For this review, take the finished solid that the model builds, in its own axes (mm). A direction names the side the tool comes from. Round coordinates to 2 decimals unless told otherwise and drop trailing zeros. Loops run counter-clockwise (first coordinate to the right, second up) from the corner with the lowest first, then second, coordinate; pieces in that order, holes last.
1) Take a section at B-B (y = 11.5). State the section outline as (x, z) points, then the cut area to 3 significant figures.
2) Insertion check: pin 1 (1.5 mm diameter, centred on x = 15.5, z = 12, fed in from -Y); pin 2 (4 mm diameter, centred on x = 34.5, y = 21, fed in from +Z); pin 3 (2 mm diameter, centred on x = 10.5, z = 24, fed in from +Y); pin 4 (7 mm diameter, centred on x = 31.02, z = 4, fed in from +Y). Each pin has a flat end and moves straight along its axis. Give the tip position at first contact, or say it passes through.
3) Take a section at C-C (z = 27). State the section outline as (x, y) points, then the cut area to 3 significant figures.
4) Tool access review of faces 4 (the flat face through (20, 58, 9)), 5 (the flat face through (19, 26, 22)), 6 (the flat face through (6.041, 31, 4)), 7 (the flat face through (9, 31, 24)): name each direction out of +Z, -Z, +X, -X, +Y, -Y from which nothing blocks a thin tool from reaching the whole face with its end or side.
5) Take a section at D-D (x = 34). State the section outline as (y, z) points.
6) Take a section at A-A (y = 26.5). Give the number of separate pieces and of enclosed holes in the cut face, then the cut area to 3 significant figures.
7) Mouldability with a two-part tool opening along X and no side actions: class faces 1 (the flat face through (7, 26, 22)), 2 (the flat face through (11, 27, 22)), 3 (the flat face through (21, 27, 34.408)) as pulls with the +X half, pulls with the -X half, needs draft (parallel to the pull), parting line crosses it, or undercut.
8) Wall thickness on L1, parallel to Z at x = 36, y = 6.5; L2, parallel to X at y = 26.5, z = 17; L3, parallel to Y at x = 1, z = 5: over which ranges is each line inside the solid? List them lowest first.
Autodesk Inventor part; units mm, degrees
ref_plane "YZ Plane" through (0, 0, 0) normal (1, 0, 0) x (0, 1, 0)
ref_plane "XZ Plane" through (0, 0, 0) normal (0, 1, 0) x (-1, 0, 0)
ref_plane "XY Plane" through (0, 0, 0) normal (0, 0, 1) x (1, 0, 0)
sketch "Sketch1" plane through (0, 0, 0) normal (0, 1, 0) x (-1, 0, 0)
  line L0 (-6.023191, 2.500092) -> (-6.023191, 5.500092) construction
  line L1 (-6.023191, 4.000092) -> (-13.023191, 4.000092) construction
  line L2 (-6.041071, 8.03122) -> (-6.041071, 4.000092)
  line L3 (-6.041071, -0.031037) -> (-13.023191, -4.062166)
  line L4 (-13.023191, -4.062166) -> (-20.005311, -0.031037)
  line L5 (-20.005311, -0.031037) -> (-20.005311, 8.03122)
  line L6 (-20.005311, 8.03122) -> (-13.023191, 12.062349)
  line L7 (-13.023191, 12.062349) -> (-6.041071, 8.03122)
  line L8 (-22.03646, 9.203905) -> (-22.03646, -1.203722)
  line L9 (-22.03646, -1.203722) -> (-13.023191, -6.407535)
  line L10 (-13.023191, 14.407718) -> (-22.03646, 9.203905)
  line L11 (-13.023191, 4.000092) -> (-31.023191, 4.000092) construction
  circle A0 centre (-31.023191, 4.000092) radius 7.5
  line L12 (-13.023191, -6.407535) -> (-30.97685, -6.407535)
  line L13 (-30.97685, -6.407535) -> (-30.97685, -3.499765)
  line L14 (-30.97685, 11.499948) -> (-30.97685, 14.407718)
  line L15 (-30.97685, 14.407718) -> (-13.023191, 14.407718)
  circle A1 centre (-13.023191, 4.000092) radius 4.5
  line L16 (-30.97685, 11.499988) -> (-30.97685, 14.407718)
  line L17 (-30.97685, -3.500012) -> (-30.97685, -6.407535)
  line L18 (-13.023191, -4.062166) -> (-13.023191, -6.407535)
  line L19 (-13.023191, 12.062349) -> (-13.023191, 14.407718)
  line L20 (-6.041071, 4.000092) -> (-6.041071, -0.031037)
  line L21 (-13.023191, 14.407718) -> (0, 14.407718)
  line L22 (0, 39) -> (0, 0)
  line L23 (0, 14.407718) -> (0, 8.03122)
  line L24 (0, 8.03122) -> (-6.041071, 8.03122)
  line L25 (0, 0) -> (-6, 0)
  line L26 (-13.023191, -6.407535) -> (-2, 0)
  line L27 (-2, 0) -> (-2, 8.03122)
  line L28 (-2, 0) -> (0, 0)
  line L29 (0, 8.03122) -> (0, 0)
  circle A2 centre (-31.023191, 4.000092) radius 4
  line L30 (-30.97685, -3.500012) -> (-38.523191, -3.500012)
  line L31 (-38.523191, -3.500012) -> (-38.523191, -6.407535)
  line L32 (-38.523191, -6.407535) -> (-30.97685, -6.407535)
  line L33 (-30.97685, -6.407535) -> (-30.97685, -3.500012)
  line L34 (-30.97685, 14.407718) -> (-38.523191, 14.407718)
  line L35 (-38.523191, 14.407718) -> (-38.523191, 11.499988)
  line L36 (-38.523191, 11.499988) -> (-30.97685, 11.499988)
  line L37 (-30.97685, 11.499988) -> (-30.97685, 14.407718)
  line L38 (0, 26) -> (-15, 26) construction
  point P0 (0, 31)
  dimension "d0" = 7
  dimension "d1" = 18
  dimension "d2" = 15
  dimension "d3" = 9
  dimension "d4" = 8
  dimension "d6" = 15
extrude "Extrusion1" add sketch "Sketch1" along normal blind 58 contours L24 L27 L26 L18 L3 L20 L2 | L7 L19 L21 L22 L24 | L6 L5 L4 L18 L9 L8 L10 L19 | L24 L22 L25 L27 | L10 L8 L9 L12 L13 A0 L14 L15 | L14 L36 L35 L34 | L32 L31 L30 L13
sketch "Sketch2" plane through (0, 0, 14.407718) normal (0, 0, 1) x (1, 0, 0)
  line L0 (0, 10) -> (15, 10) construction
  line L1 (0, 0) -> (38.523191, 0) construction
  line L2 (15, 0) -> (15, 6.5) construction
  line L3 (15, 0) -> (21.5, 0) construction
  circle A0 centre (15, 6.5) radius 4
  line L4 (15, 6.5) -> (15, 46.5) construction
  line L5 (23.523191, 58) -> (23.523191, 0) construction
  line L6 (15, 6.5) -> (55, 6.5) construction
  circle A1 centre (15, 46.5) radius 4
  circle A2 centre (15, 46.5) radius 6.576473
  circle A3 centre (15, 6.5) radius 6.726812
  line L7 (15, 46.5) -> (15, 26.5) construction
  line L8 (15, 46.5) -> (35, 46.5) construction
  line L9 (15, 26.5) -> (11, 26.5) construction
  line L10 (15, 26.5) -> (19, 26.5) construction
  line L11 (15, 26.5) -> (19, 26.5) construction
  line L12 (7, 31) -> (11, 31)
  line L13 (11, 31) -> (11, 22)
  line L14 (11, 22) -> (7, 22)
  line L15 (7, 22) -> (7, 31)
  line L16 (7, 31) -> (11, 22) construction
  line L17 (11, 31) -> (7, 22) construction
  line L18 (23, 22) -> (19, 22)
  line L19 (19, 22) -> (19, 31)
  line L20 (19, 31) -> (23, 31)
  line L21 (23, 31) -> (23, 22)
  line L22 (23, 22) -> (19, 31) construction
  line L23 (19, 22) -> (23, 31) construction
  point P0 (9, 26.5)
  point P1 (21, 26.5)
  dimension "d9" = 15
  dimension "d10" = 6.5
  dimension "d11" = 90
  dimension "d12" = 8
  dimension "d13" = 40
  dimension "d14" = 90
  dimension "d15" = 8
  dimension "d16" = 2.57647
  dimension "d17" = 2.72681
  dimension "d18" = 20
  dimension "d19" = 90
  dimension "d20" = 4
  dimension "d21" = 180
extrude "Extrusion2" add sketch "Sketch2" along normal blind 15 contours A2 | A3
extrude "Extrusion3" add sketch "Sketch2" along normal blind 20 contours L12 L13 L14 L15 | L18 L19 L20 L21
hole "Hole1" at (7, 26.5, 28.407718) direction (1, 0, 0) diameter 8 end through all
extrude "Extrusion4" add sketch "Sketch1" along normal blind 4 contours L2 L20 L3 L4 L5 L6 L7
hole "Hole2" at (0, 53, 5) direction (1, 0, 0) diameter 4 end up to surface
sketch "Sketch1 outline for Extrusion5" plane through (0, 0, 0) normal (0, 1, 0) x (-1, 0, 0)
  arc A0 (-30.97685, 11.499948) -> (-30.97685, -3.499765) centre (-31.023191, 4.000092) ccw
  arc A1 (-30.97685, -3.499765) -> (-30.97685, 11.499948) centre (-31.023191, 4.000092) ccw
  circle A2 centre (-31.023191, 4.000092) radius 4
extrude "Extrusion5" add sketch "Sketch1 outline for Extrusion5" along normal blind 2
properties part number "XMountR"
Response:
1. outline: (0, 0) - (2, 0) - (13.02, -6.41) - (38.52, -6.41) - (38.52, -3.5) - (30.98, -3.5) arc R7.5 cw to (30.98, 11.5) - (38.52, 11.5) - (38.52, 14.41) - (19.5, 14.41) - (19.5, 29.41) - (10.5, 29.41) - (10.5, 14.41) - (0, 14.41) - close; hole (6.04, -0.03) - (13.02, -4.06) - (20.01, -0.03) - (20.01, 8.03) - (13.02, 12.06) - (6.04, 8.03) - close
1. area: 519 mm2
2. pin 1: stops at y = 0
2. pin 2: stops at z = 14.41
2. pin 3: stops at y = 52.07
2. pin 4: passes through
3. outline: (7, 22) - (11, 22) - (11, 22.76) - (7, 22.76) - close; (7, 30.24) - (11, 30.24) - (11, 31) - (7, 31) - close; circle Ø13.45 at (15, 6.5); circle Ø13.15 at (15, 46.5); (19, 22) - (23, 22) - (23, 22.76) - (19, 22.76) - close; (19, 30.24) - (23, 30.24) - (23, 31) - (19, 31) - close; hole circle Ø8 at (15, 6.5); hole circle Ø8 at (15, 46.5)
3. area: 190 mm2
4. face 4: +Z, -Z, +X, -X, +Y
4. face 5: +Z
4. face 6: +Y
4. face 7: +Z, +X, -X
5. outline: (0, -6.41) - (58, -6.41) - (58, -3.5) - (0, -3.5) - close; (0, -2.88) - (2, -2.88) - (2, 1.33) - (0, 1.33) - close; (0, 6.67) - (2, 6.67) - (2, 10.88) - (0, 10.88) - close; (0, 11.5) - (58, 11.5) - (58, 14.41) - (0, 14.41) - close
6. separate pieces: 3
6. enclosed holes: 1
6. area: 480 mm2
7. face 1: pulls with the -X half
7. face 2: undercut
7. face 3: needs draft
8. L1: z = -6.41 to -3.5, 11.5 to 14.41
8. L2: x = 7 to 11, 19 to 23
8. L3: y = 0 to 51, 55 to 58
